from build123d import *

# Parameters (mm, degrees)
F0_W     = 50
F0_H     = 30
F1_DEPTH = 0.45


with BuildPart() as f1:
    # F0 (on Top) → F1 (new body)
    with BuildSketch(Plane.XY):
        with Locations((25, 15)):
            Rectangle(F0_W, F0_H)
        with BuildLine():
            Line((50, 30), (50, 0))
            ThreePointArc((50, 0), (60, 15), (50, 30))
        make_face()
    extrude(amount=F1_DEPTH)


with BuildPart() as f2_1:
    # F2: copy of F1
    add(f1.part)


solid = f1.part
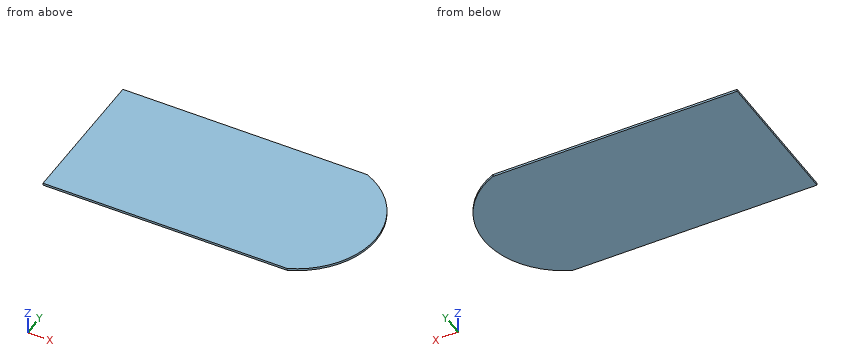
The model under review builds one solid part; all positions refer to its coordinate system, in mm. Round coordinates to 2 decimals unless told otherwise and drop trailing zeros. Loops run counter-clockwise (first coordinate to the right, second up) from the corner with the lowest first, then second, coordinate; pieces in that order, holes last. Notation, with made-up numbers: (-21, -18.75) -> (-2, -18.75) arc R11 ccw to (-2, -8.75) -> close; hole circle Ø6 at (7.25, 57.5). An arc over 180 degrees is marked (long way). Return JSON: item names as keys, results as strings.
(1) Add section A-A on z = 0.1. Write out the cut boundary in (x, y).
Solved:
{"outline": "(0, 0) -> (50, 0) arc R16.25 ccw to (50, 30) -> (0, 30) -> close"}
(2) For line 1 (X direction, y = 9.5, z = 0.3); line 2 (Y direction, x = 50.5, z = 0.25); line 3 (X direction, y = 12.25, z = 0.2), list the stretches that pass through material, from the lowest coordinate up.
Solved:
{"line 1": "0 to 59.04", "line 2": "0.22 to 29.78", "line 3": "0 to 59.77"}
(3) Add section B-B on y = 28. Write out the cut boundary in (x, z), plus the area to 3 significant figures.
Solved:
{"outline": "(0, 0) -> (53.5, 0) -> (53.5, 0.45) -> (0, 0.45) -> close", "area": "24.1 mm2"}
